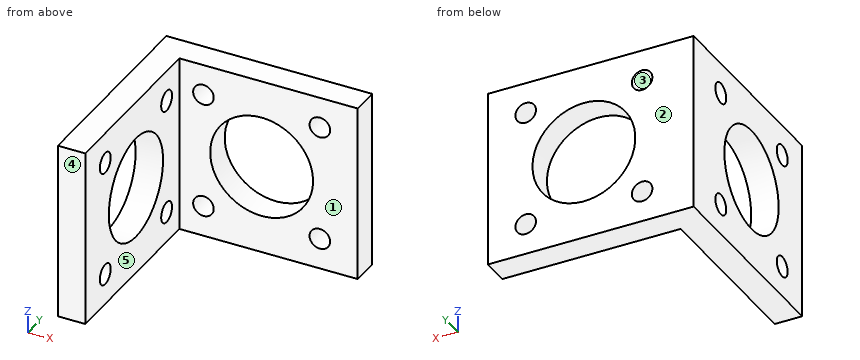
Autodesk Inventor part; units mm, degrees
ref_plane "YZ Plane" through (0, 0, 0) normal (1, 0, 0) x (0, 1, 0)
ref_plane "XZ Plane" through (0, 0, 0) normal (0, 1, 0) x (-1, 0, 0)
ref_plane "XY Plane" through (0, 0, 0) normal (0, 0, 1) x (1, 0, 0)
ref_plane "Work Plane1" through (-18.4246, 0, 0) normal (0, 0, 1) x (1, 0, 0)
sketch "Sketch1" plane through (-18.4246, 0, 0) normal (0, 0, 1) x (1, 0, 0)
  line L0 (0, -0.9373) -> (0, 15)
  line L1 (0, 15) -> (15.9373, 15)
  line L2 (0, -0.9373) -> (0, 19.0627)
  line L3 (15.9373, 15) -> (-4.0627, 15)
  line L4 (0, 15) -> (2, 15)
  line L5 (2, 15) -> (2, 0)
  line L6 (2, 0) -> (0, 0)
  line L7 (0, 0) -> (0, 15)
  line L8 (0, 15) -> (15, 15)
  line L9 (15, 15) -> (15, 13)
  line L10 (15, 13) -> (0, 13)
  line L11 (0, 13) -> (0, 15)
  point P0 (18.4246, 0)
  point P1 (0, 0)
  point P2 (2, 13)
  point P3 (15, 15)
  dimension "d0" = 20
  dimension "d1" = 20
  dimension "d2" = 2
  dimension "d3" = 15
  dimension "d4" = 15
  dimension "d5" = 2
extrude "Extrusion1" add sketch "Sketch1" along normal blind 13
sketch "Sketch2" plane through (-16.4246, 0, 0) normal (1, 0, 0) x (0, 0, -1)
  circle A0 centre (-10.7426, 2.7574) radius 0.75
  circle A1 centre (-10.7426, 11.2426) radius 0.75
  circle A2 centre (-2.2574, 2.7574) radius 0.75
  circle A3 centre (-2.2574, 11.2426) radius 0.75
  point P0 (0, 0)
extrude "Extrusion2" cut sketch "Sketch2" against normal blind 13
sketch "Sketch3" plane through (-16.4246, 13, 0) normal (0, -1, 0) x (1, 0, 0)
  circle A0 centre (1.7574, 10.7426) radius 0.75
  circle A1 centre (10.2426, 10.7426) radius 0.75
  circle A2 centre (10.2426, 2.2574) radius 0.75
  circle A3 centre (1.7574, 2.2574) radius 0.75
  point P0 (16.4246, 0)
extrude "Extrusion3" cut sketch "Sketch3" against normal blind 13
sketch "Sketch4" plane through (-16.4246, 0, 0) normal (1, 0, 0) x (0, 0, -1)
  point P0 (0, 0)
sketch "Sketch5" plane through (-16.4246, 0, 0) normal (1, 0, 0) x (0, 0, -1)
  circle A0 centre (-6.5, 7) radius 1.5
  circle A1 centre (-6.5, 7) radius 3.75
  point P0 (0, 0)
  dimension "d12" = 7.5
extrude "Extrusion4" cut sketch "Sketch5" against normal blind 13 contours A0 | A1
sketch "Sketch6" plane through (-16.4246, 13, 0) normal (0, -1, 0) x (1, 0, 0)
  circle A0 centre (6, 6.5) radius 1.5
  circle A1 centre (6, 6.5) radius 3.75
  point P0 (16.4246, 0)
  dimension "d15" = 7.5
extrude "Extrusion5" cut sketch "Sketch6" against normal blind 13 contours A0 | A1
properties part number "base_1"
Here's how the part is built. I have some questions about the finished solid (model axes, mm). Face numbers are marked on the shaded views. A direction names the side the tool comes from. Give positions to 0.01 mm unless a question says otherwise; leave off trailing zeros. Loops run counter-clockwise (first coordinate to the right, second up) from the corner with the lowest first, then second, coordinate; pieces in that order, holes last. Notation, with made-up numbers: (53, 33) -> (71, 33) arc R13 cw to (71, 48) -> close; hole circle Ø7 at (-13, 28.5). An arc over 180 degrees is marked (long way). Use one line per item in the form item = value. Start each with the question number.
1) Imagine slicing it at A-A (z = 6.5). Please give me the cut outline in (x, y).
2) Imagine slicing it at C-C (x = -11). Please give me the cut outline in (y, z), then the cut area to 3 significant figures.
3) Please list where these lines run through material, in increasing order: line 1 along Y through (x, z) = (-4.5, 5.25); line 2 along Z through (x, y) = (-7.75, 14.25); line 3 along X through (y, z) = (3.5, 12.25).
4) Imagine slicing it at B-B (y = 7). Please give me the cut outline in (x, z).
5) Imagine slicing it at D-D (y = 11). Please give me the cut outline in (x, z), then the cut area to 3 significant figures.
6) Which directions (+Z, -Z, +X, -X, +Y, -Y) give clear straight access to the entire face, cutting with the end or side of a thin tool? Please do the marked faces 1 and 2.
7) Thinking about a two-plate mould opening in X: for the marked faces 3, 4 and 5, which applies, +X half, -X half, draft (parallel to the pull), parting line (faces both ways), or undercut?
8) For P1, Ø1.7, axis at x = -14.67, z = 10.74, coming from the +Y side; P2, Ø6.5, axis at y = 9.5, z = 4, coming from the +X side; P3, Ø1.7, axis at x = -6.18, z = 2.26, coming from the -Y side, each with a flat end and sliding along its axis, tell me the tip position at first contact or that it passes through.
Check values:
q1.outline = (-18.42, 0) -> (-16.42, 0) -> (-16.42, 3.25) -> (-18.42, 3.25) -> close; (-18.42, 10.75) -> (-16.42, 10.75) -> (-16.42, 13) -> (-14.17, 13) -> (-14.17, 15) -> (-18.42, 15) -> close; (-6.67, 13) -> (-3.42, 13) -> (-3.42, 15) -> (-6.67, 15) -> close
q2.outline = (13, 0) -> (15, 0) -> (15, 2.79) -> (13, 2.79) -> close; (13, 10.21) -> (15, 10.21) -> (15, 13) -> (13, 13) -> close
q2.area = 11.2 mm^2
q3.line_1 = 13 to 15
q3.line_2 = 0 to 3.87, 9.13 to 13
q3.line_3 = -18.42 to -16.42
q4.outline = (-18.42, 0) -> (-16.42, 0) -> (-16.42, 2.75) -> (-18.42, 2.75) -> close; (-18.42, 10.25) -> (-16.42, 10.25) -> (-16.42, 13) -> (-18.42, 13) -> close
q5.outline = (-18.42, 0) -> (-16.42, 0) -> (-16.42, 1.55) -> (-18.42, 1.55) -> close; (-18.42, 2.97) -> (-16.42, 2.97) -> (-16.42, 10.03) -> (-18.42, 10.03) -> close; (-18.42, 11.45) -> (-16.42, 11.45) -> (-16.42, 13) -> (-18.42, 13) -> close
q5.area = 20.3 mm^2
q6.face_1 = +Z, -Z, +X, -Y
q6.face_2 = +Z, -Z, +X, -X, +Y
q7.face_3 = undercut
q7.face_4 = draft
q7.face_5 = +X half
q8.P1 = 15
q8.P2 = -16.42
q8.P3 = 13
